Design review of the part built by this model. Coordinates are the model's own, in mm. A direction names the side the tool comes from. Give positions to 0.01 mm unless a question says otherwise; leave off trailing zeros. Loops run counter-clockwise (first coordinate to the right, second up) from the corner with the lowest first, then second, coordinate; pieces in that order, holes last.
from build123d import *
from build123d.topology import SkipClean

# Parameters (mm, degrees)
BOSS_EXTRUDE1_DEPTH     = 24
CUT_EXTRUDE1_DEPTH      = 91.21363533302491
CUT_EXTRUDE1_DEPTH_BACK = 91.21363533302491
SKETCH2_4_R             = 16.25
CUT_EXTRUDE2_DEPTH      = 3
CUT_EXTRUDE2_DEPTH_BACK = 48
SKETCH2_5_R             = 19.5
SKETCH2_5_R_2           = 16.25
CUT_EXTRUDE3_DEPTH      = 48
CUT_EXTRUDE3_DEPTH_BACK = 16
SKETCH3_W               = 8.5
SKETCH3_H               = 14.200000000000006
CUT_EXTRUDE4_DEPTH      = 40
SKETCH7_R               = 27.499999999999996
SKETCH7_R_2             = 18.9
BOSS_EXTRUDE2_DEPTH     = 1
SKETCH8_W               = 181.3602376825947
SKETCH8_H               = 155.21218123297842
CUT_EXTRUDE5_DEPTH      = 48
BOSS_EXTRUDE3_START     = 48
SKETCH9_R               = 27.499999999999996
SKETCH9_R_2             = 18.9
BOSS_EXTRUDE3_DEPTH     = 48
CUT_EXTRUDE6_DEPTH      = 48
BOSS_EXTRUDE4_DEPTH     = 4
EXTRUDE_THIN2_DEPTH     = 30
CUT_EXTRUDE8_START      = -21
CUT_EXTRUDE8_DEPTH      = 21
BOSS_EXTRUDE5_DEPTH     = 21
CUT_EXTRUDE9_DEPTH      = 21
CUT_EXTRUDE10_DEPTH     = 5
SKETCH21_R              = 27.499999999999996
SKETCH21_R_2            = 7.25
BOSS_EXTRUDE6_DEPTH     = 3


with BuildPart() as part:
    # Sketch2 → Boss-Extrude1 (new, symmetric)
    with BuildSketch(Plane.XY):
        with BuildLine():
            ThreePointArc((-24.69493875270801, -42.900000000000006), (1.68e-15, -82.5), (24.694938752708016, -42.9))
            ThreePointArc((24.694938752708016, -42.9), (21.124860801609124, -27.49999999999999), (24.694938752708012, -12.099999999999996))
            ThreePointArc((24.694938752708012, -12.099999999999996), (3.42e-15, 27.499999999999996), (-24.694938752708012, -12.100000000000001))
            ThreePointArc((-24.694938752708012, -12.100000000000001), (-21.124860801609117, -27.500000000000004), (-24.69493875270801, -42.900000000000006))
        make_face()
    extrude(amount=BOSS_EXTRUDE1_DEPTH, both=True)

    # Sketch2<4> → Cut-Extrude1 (cut, two sides: drawn at the far end of the back side and taken through both)
    with BuildSketch(Plane.XY.offset(-CUT_EXTRUDE1_DEPTH_BACK)):
        with Locations((6.74e-15, -55)):
            Circle(SKETCH2_4_R)
    extrude(amount=CUT_EXTRUDE1_DEPTH + CUT_EXTRUDE1_DEPTH_BACK, mode=Mode.SUBTRACT)

    # Sketch2<5> → Cut-Extrude2 (cut, two sides: drawn at the far end of the back side and taken through both)
    with BuildSketch(Plane.XY.offset(-CUT_EXTRUDE2_DEPTH_BACK)):
        with Locations((6.74e-15, -55)):
            Circle(SKETCH2_5_R)
        with Locations((6.74e-15, -55)):
            Circle(SKETCH2_5_R_2, mode=Mode.SUBTRACT)
    extrude(amount=CUT_EXTRUDE2_DEPTH + CUT_EXTRUDE2_DEPTH_BACK, mode=Mode.SUBTRACT)

    # Sketch2<6> → Cut-Extrude3 (cut, two sides: drawn at the far end of the back side and taken through both)
    with BuildSketch(Plane.XY.offset(-CUT_EXTRUDE3_DEPTH_BACK)):
        Polygon((10.399999999999997, 20.400000000000002), (-10.400000000000002, 20.400000000000002), (-10.399999999999999, -20.399999999999995), (10.400000000000002, -20.399999999999995), align=None)
    extrude(amount=CUT_EXTRUDE3_DEPTH + CUT_EXTRUDE3_DEPTH_BACK, mode=Mode.SUBTRACT)

    # Sketch3 → Cut-Extrude4 (cut)
    with BuildSketch(Plane.XY.offset(24)):
        with Locations((0, 27.500000000000007)):
            Rectangle(SKETCH3_W, SKETCH3_H)
    extrude(amount=-CUT_EXTRUDE4_DEPTH, mode=Mode.SUBTRACT)

    # Sketch7 → Boss-Extrude2 (add)
    with BuildSketch(Plane(origin=(0, 0, -24), x_dir=(-1, 0, 0), z_dir=(0, 0, -1))):
        with Locations((-6.74e-15, -55)):
            Circle(SKETCH7_R)
        with Locations((-6.74e-15, -55)):
            Circle(SKETCH7_R_2, mode=Mode.SUBTRACT)
    extrude(amount=BOSS_EXTRUDE2_DEPTH)

    # Sketch8 → Cut-Extrude5 (cut)
    with BuildSketch(Plane.XY.offset(24)):
        with Locations((-25.06580059332441, -26.494305521168478)):
            Rectangle(SKETCH8_W, SKETCH8_H)
    extrude(amount=-CUT_EXTRUDE5_DEPTH, mode=Mode.SUBTRACT)

    # Sketch9 → Boss-Extrude3 (add)
    with SkipClean():  # the faces are left unmerged after this step: merging them gives an invalid solid
        with BuildSketch(Plane.XY.offset(-24).offset(BOSS_EXTRUDE3_START)):
            with Locations(Location((6.74e-15, -55, 0), (0, 0, 180))):
                Circle(SKETCH9_R)
            with Locations((6.74e-15, -55)):
                Circle(SKETCH9_R_2, mode=Mode.SUBTRACT)
        extrude(amount=-BOSS_EXTRUDE3_DEPTH)

    # Sketch10 → Cut-Extrude6 (cut)
    with SkipClean():  # the faces are left unmerged after this step: merging them gives an invalid solid
        with BuildSketch(Plane.XY.offset(24)):
            with BuildLine():
                Line((26.717930940571712, -48.48830542371335), (26.510281823927063, -55))
                Line((26.510281823927063, -55), (26.510281823927063, -62.311289736835946))
                ThreePointArc((26.51028182392707, -62.311289736835946), (27.25144721072622, -58.68898697761363), (27.500000000000014, -55))
                ThreePointArc((27.500000000000014, -55), (27.30378271289276, -51.72075472598662), (26.717930940571723, -48.48830542371334))
            make_face()
            with BuildLine():
                ThreePointArc((-5.604082705298323, -81.92293180603063), (6e-15, -82.5), (5.604082705298339, -81.92293180603063))
                Line((5.604082705298337, -81.92293180603063), (6.74e-15, -81.92293180603063))
                Line((7.11e-15, -81.92293180603063), (-5.604082705298323, -81.92293180603063))
            make_face()
        extrude(amount=-CUT_EXTRUDE6_DEPTH, mode=Mode.SUBTRACT)

    # Sketch11 → Boss-Extrude4 (add)
    with SkipClean():  # the faces are left unmerged after this step: merging them gives an invalid solid
        with BuildSketch(Plane.XY.offset(24)):
            with BuildLine():
                ThreePointArc((27.500000000000025, -55.00000000000003), (27.300326018506244, -58.3078995273848), (26.7042036884893, -61.56776258429582))
                Line((26.70420368848926, -61.56776258429563), (42.21724684134985, -61.56776258429563))
                Line((42.21724684134985, -61.56776258429563), (42.21724684134985, 29.98869686217629))
                Line((42.21724684134985, 29.988696862176287), (-3.7193423220770256, 29.988696862176287))
                Line((-3.719342322077025, 29.988696862176287), (-3.719342322077025, -27.7526791648939))
                ThreePointArc((-3.719342322077028, -27.7526791648939), (15.483065545848751, -32.27282064789051), (26.717930940571723, -48.488305423713314))
                ThreePointArc((26.717930940571723, -48.488305423713314), (27.303782712892772, -51.72075472598662), (27.500000000000025, -55.00000000000002))
            make_face()
        extrude(amount=-BOSS_EXTRUDE4_DEPTH)

    # Sketch16 → Extrude-Thin2 (add)
    with SkipClean():  # the faces are left unmerged after this step: merging them gives an invalid solid
        with BuildSketch(Plane(origin=(0, 0, 24), x_dir=(-1, 0, 0), z_dir=(0, 0, -1))):
            with BuildLine():
                Line((-26.704203688489347, -61.56776258429563), (-42.21724684134985, -61.56776258429563))
                Line((-42.21724684134985, -61.56776258429563), (-42.21724684134985, 29.988696862176287))
                Line((-42.21724684134985, 29.988696862176287), (3.719342322077025, 29.988696862176287))
                Line((3.719342322077025, 29.988696862176287), (3.719342322077025, -27.75267916489391))
                ThreePointArc((3.719342322077025, -27.75267916489391), (-20.443603637167037, -36.60682000505511), (-26.704203688489347, -61.56776258429563))
            make_face()
            with BuildLine():
                Line((-29.722942444479006, -59.06776258429563), (-39.71724684134985, -59.06776258429563))
                Line((-39.71724684134985, -59.06776258429563), (-39.71724684134985, 27.48869686217629))
                Line((-39.71724684134985, 27.48869686217629), (1.2193423220770256, 27.488696862176287))
                Line((1.2193423220770256, 27.488696862176287), (1.2193423220770252, -25.02479017084956))
                ThreePointArc((1.2193423220770252, -25.02479017084956), (-22.200108055370485, -34.82191281786335), (-29.722942444479006, -59.06776258429563))
            make_face(mode=Mode.SUBTRACT)
        extrude(amount=EXTRUDE_THIN2_DEPTH)

    # Sketch17 → Cut-Extrude8 (cut)
    with BuildSketch(Plane(origin=(0, 0, -5.999999999999998), x_dir=(-1, 0, 0), z_dir=(0, 0, -1)).offset(CUT_EXTRUDE8_START)):
        with BuildLine():
            Line((1.3487027041970006, -27.53309262010562), (1.2193423220770252, -25.02479017084956))
            ThreePointArc((1.2193423220770252, -25.02479017084956), (-22.20010805537015, -34.82191281786366), (-29.72294244447902, -59.06776258429561))
            Line((-29.72294244447902, -59.06776258429561), (-27.19748715520997, -59.06776258429561))
            ThreePointArc((-27.19748715520997, -59.06776258429561), (-20.38746592483553, -36.54461506324843), (1.3487027041970006, -27.53309262010562))
        make_face()
    extrude(amount=CUT_EXTRUDE8_DEPTH, mode=Mode.SUBTRACT)

    # Sketch18 → Boss-Extrude5 (add)
    with BuildSketch(Plane(origin=(0, 0, 20), x_dir=(-1, 0, 0), z_dir=(0, 0, -1))):
        with BuildLine():
            ThreePointArc((-27.19748715520984, -50.93223741570337), (-17.949742740939968, -34.16597169210712), (-1.0275e-13, -27.499999999999904))
            Line((-1.0275e-13, -27.499999999999908), (-11.98957880828152, -27.499999999999908))
            ThreePointArc((-11.98957880828161, -27.49999999999943), (-20.951294804022364, -33.528082385707165), (-27.197487155209934, -42.33916699256241))
            Line((-27.197487155209956, -42.339166992562404), (-27.197487155209956, -50.93223741570336))
        make_face()
    extrude(amount=BOSS_EXTRUDE5_DEPTH)

    # Sketch19 → Cut-Extrude9 (cut)
    with BuildSketch(Plane(origin=(0, 0, -5.999999999999998), x_dir=(-1, 0, 0), z_dir=(0, 0, -1))):
        Polygon((-39.71724684134985, 27.48869686217629), (-39.71724684134984, 29.988696862176287), (-19.248952259636408, 29.988696862176287), (-19.24895225963641, 27.48869686217629), align=None)
    extrude(amount=-CUT_EXTRUDE9_DEPTH, mode=Mode.SUBTRACT)

    # Sketch20 → Cut-Extrude10 (cut)
    with BuildSketch(Plane(origin=(0, 0, 15.000000000000004), x_dir=(-1, 0, 0), z_dir=(0, 0, -1))):
        Polygon((-19.248952259636408, 29.988696862176287), (-39.71724684134984, 29.988696862176287), (-39.71724684134984, 27.48869686217629), (-19.24895225963641, 27.48869686217629), align=None)
    extrude(amount=-CUT_EXTRUDE10_DEPTH, mode=Mode.SUBTRACT)

    # Sketch21 → Boss-Extrude6 (add)
    with BuildSketch(Plane.XY.offset(24)):
        with Locations(Location((6.74e-15, -55, 0), (0, 0, 180))):
            Circle(SKETCH21_R)
        with Locations((6.74e-15, -55)):
            Circle(SKETCH21_R_2, mode=Mode.SUBTRACT)
    extrude(amount=-BOSS_EXTRUDE6_DEPTH)


solid = part.part
Q1. Insertion check: pin 1 (16.5 mm diameter, centred on x = 10, z = 3.5, fed in from -Y); pin 2 (6.5 mm diameter, centred on x = 34, z = 6.5, fed in from +Y); pin 3 (1 mm diameter, centred on y = -56, z = -14.5, fed in from +X); pin 4 (18.5 mm diameter, centred on x = 8, y = -40, fed in from -Z). Each pin has a flat end and moves straight along its axis. Give the tip position at first contact, or say it passes through.
Results:
pin 1: stops at y = -81.92
pin 2: stops at y = -59.07
pin 3: stops at x = 26.51
pin 4: stops at z = -25
Q2. Take a section at A-A (z = 11). Give the boundary of the cut face in (x, y), plus the area to 3 significant figures.
Results:
outline: (-5.6, -81.92) - (5.6, -81.92) arc R27.5 ccw to (26.51, -62.31) - (26.51, -55) - (26.72, -48.49) arc R27.5 cw to (27.2, -50.93) - (27.2, -42.34) arc R30 ccw to (11.99, -27.5) - (0, -27.5) arc R27.5 ccw to (-1.35, -27.53) - (-1.22, -25.02) - (-1.22, 27.49) - (19.25, 27.49) - (19.25, 29.99) - (-3.72, 29.99) - (-3.72, -27.75) arc R27.5 ccw to start; (26.7, -61.57) - (42.22, -61.57) - (42.22, 29.99) - (39.72, 29.99) - (39.72, -59.07) - (27.2, -59.07) arc R27.5 cw to start; hole circle Ø37.8 at (0, -55)
area: 1,770 mm2
Q3. Wall thickness on line 1 (X direction, y = -55, z = -2); line 2 (X direction, y = 25, z = -5.5); line 3 (Y direction, x = 0, z = 7): over which ranges is each line inside the solid? List them lowest first.
Results:
line 1: x = -27.5 to -18.9, 18.9 to 26.51, 39.72 to 42.22
line 2: x = -3.72 to -1.22, 39.72 to 42.22
line 3: y = -81.92 to -73.9, -36.1 to -27.5, 27.49 to 29.99
Q4. Draft analysis for pull direction X (two halves, no side actions). For faces 1 (the face through (-3.719, 2, 9)), 2 (the face through (34, -61.568, 9)), 3 (the face through (3.35, -61.43, 22.52)), state which applies: pulls with the +X half, pulls with the -X half, needs draft (parallel to the pull), parting line crosses it, or undercut.
Results:
face 1: pulls with the -X half
face 2: needs draft
face 3: undercut
Q5. Take a section at C-C (x = 36). Give the boundary of the cut face in (y, z), plus the area to 3 significant figures.
Results:
outline: (-61.57, -6) - (-59.07, -6) - (-59.07, 20) - (29.99, 20) - (29.99, 24) - (-61.57, 24) - close
area: 431 mm2
Q6. Take a section at D-D (z = -8). Give the boundary of the cut face in (x, y).
Results:
outline: (-5.6, -81.92) - (5.6, -81.92) arc R27.5 ccw to (26.51, -62.31) - (26.51, -55) - (26.72, -48.49) arc R27.5 ccw (long way) to start; hole circle Ø37.8 at (0, -55)
Q7. Take a section at B-B (y = 23.5). Give the boundary of the cut face in (x, z).
Results:
outline: (-3.72, -6) - (-1.22, -6) - (-1.22, 20) - (39.72, 20) - (39.72, -6) - (42.22, -6) - (42.22, 24) - (-3.72, 24) - close
Q8. Tool access review of faces 4 (the face through (29, -52, 15)), 5 (the face through (27.16, -59.32, 10.69)), 6 (the face through (6, -27.5, 7)), 7 (the face through (26.51, -59, -1)), 8 (the face through (40, -22, -6)): name each direction out of +Z, -Z, +X, -X, +Y, -Y from which nothing blocks a thin tool from reaching the whole face with its end or side.
Results:
face 4: -Z, +Y
face 5: none
face 6: -Z
face 7: -Y
face 8: -Z, +X, +Y, -Y
